from build123d import *

# Parameters (mm, degrees)
F0_W     = 60.086440295
F0_H     = 106.3739694655
F1_DEPTH = 25.4
F3_DEPTH = 12.7
F4_R     = 8.89
F4_R_2   = 5.08
F5_DEPTH = 15.24
F7_DEPTH = 12.7


with BuildPart() as f1:
    # F0 (on Top) → F1 (new body)
    with BuildSketch(Plane.XY):
        with Locations((-30.0432201475, -10.3531312197)):
            Rectangle(F0_W, F0_H)
    extrude(amount=F1_DEPTH)

    # F2 (on face) → F3 (join)
    with BuildSketch(Plane.XY.offset(25.4)):
        with BuildLine():
            ThreePointArc((-10.16, -38.1401159525), (-25.3361792847, -31.8539366677), (-19.05, -47.0301159525))
            Line((-19.05, -47.0301159525), (-19.05, -38.1401159525))
            Line((-19.05, -38.1401159525), (-10.16, -38.1401159525))
        make_face()
        with BuildLine():
            Line((-19.05, -38.1401159525), (-19.05, -47.0301159525))
            ThreePointArc((-19.05, -47.0301159525), (-12.7638207153, -44.4262952372), (-10.16, -38.1401159525))
            Line((-10.16, -38.1401159525), (-19.05, -38.1401159525))
        make_face()
        with BuildLine():
            ThreePointArc((-49.926440295, -38.1401159525), (-47.3226195797, -44.4262952372), (-41.036440295, -47.0301159525))
            Line((-41.036440295, -47.0301159525), (-41.036440295, -38.1401159525))
            Line((-41.036440295, -38.1401159525), (-49.926440295, -38.1401159525))
        make_face()
        with BuildLine():
            Line((-41.036440295, -38.1401159525), (-41.036440295, -47.0301159525))
            ThreePointArc((-41.036440295, -47.0301159525), (-34.7502610102, -44.4262952372), (-32.146440295, -38.1401159525))
            ThreePointArc((-32.146440295, -38.1401159525), (-41.036440295, -29.2501159525), (-49.926440295, -38.1401159525))
            Line((-49.926440295, -38.1401159525), (-41.036440295, -38.1401159525))
        make_face()
        with BuildLine():
            ThreePointArc((-41.036440295, 26.323853513), (-47.3226195797, 23.7200327978), (-49.926440295, 17.433853513))
            Line((-49.926440295, 17.433853513), (-41.036440295, 17.433853513))
            Line((-41.036440295, 17.433853513), (-41.036440295, 26.323853513))
        make_face()
        with BuildLine():
            Line((-41.036440295, 17.433853513), (-49.926440295, 17.433853513))
            ThreePointArc((-49.926440295, 17.433853513), (-41.036440295, 8.543853513), (-32.146440295, 17.433853513))
            ThreePointArc((-32.146440295, 17.433853513), (-34.7502610102, 23.7200327978), (-41.036440295, 26.323853513))
            Line((-41.036440295, 26.323853513), (-41.036440295, 17.433853513))
        make_face()
        with BuildLine():
            ThreePointArc((-19.05, 26.323853513), (-25.9314853388, 11.8055980522), (-10.3366687432, 15.6703460962))
            ThreePointArc((-10.3366687432, 15.6703460962), (-10.2042774497, 16.5476861679), (-10.16, 17.433853513))
            ThreePointArc((-10.16, 17.433853513), (-12.7638207153, 23.7200327978), (-19.05, 26.323853513))
        make_face()
    extrude(amount=F3_DEPTH)

    # F4 (on face) → F5 (join)
    with BuildSketch(Plane.XY.offset(25.4)):
        with Locations((-41.036440295, -38.1401159525)):
            Circle(F4_R)
        with Locations((-41.036440295, -38.1401159525)):
            Circle(F4_R_2, mode=Mode.SUBTRACT)
        with Locations((-19.05, -38.1401159525)):
            Circle(F4_R)
        with Locations((-19.05, -38.1401159525)):
            Circle(F4_R_2, mode=Mode.SUBTRACT)
        with Locations((-41.036440295, 17.433853513)):
            Circle(F4_R)
        with Locations((-41.036440295, 17.433853513)):
            Circle(F4_R_2, mode=Mode.SUBTRACT)
        with Locations((-19.05, 17.433853513)):
            Circle(F4_R)
        with Locations((-19.05, 17.433853513)):
            Circle(F4_R_2, mode=Mode.SUBTRACT)
    extrude(amount=F5_DEPTH)

    # F6 (on face) → F7 (cut)
    with BuildSketch(Plane(origin=(0, 0, 0), x_dir=(1, 0, 0), z_dir=(0, 0, -1))):
        with BuildLine():
            Line((-53.6326494753, 38.1401159525), (-48.3460910618, 38.1401159525))
            Line((-48.3460910618, 38.1401159525), (-48.3460910618, 46.6701357601))
            ThreePointArc((-48.3460910618, 46.6701357601), (-52.20384553, 43.1578080957), (-53.6326494753, 38.1401159525))
        make_face()
        with BuildLine():
            Line((-34.5826494753, 38.1401159525), (-48.3460910618, 38.1401159525))
            Line((-48.3460910618, 38.1401159525), (-53.6326494753, 38.1401159525))
            ThreePointArc((-53.6326494753, 38.1401159525), (-44.1076494753, 28.6151159525), (-34.5826494753, 38.1401159525))
        make_face()
        with BuildLine():
            Line((-48.3460910618, 46.6701357601), (-48.3460910618, 38.1401159525))
            Line((-48.3460910618, 38.1401159525), (-34.5826494753, 38.1401159525))
            ThreePointArc((-34.5826494753, 38.1401159525), (-39.0899573321, 46.2363120072), (-48.3460910618, 46.6701357601))
        make_face()
        with BuildLine():
            Line((-7.6825144947, 38.1401159525), (-26.7325144947, 38.1401159525))
            ThreePointArc((-26.7325144947, 38.1401159525), (-17.2075144947, 28.6151159525), (-7.6825144947, 38.1401159525))
        make_face()
        with BuildLine():
            ThreePointArc((-7.6825144947, 38.1401159525), (-17.2075144947, 47.6651159525), (-26.7325144947, 38.1401159525))
            Line((-26.7325144947, 38.1401159525), (-7.6825144947, 38.1401159525))
        make_face()
        with BuildLine():
            ThreePointArc((-26.7325144947, -17.433853513), (-17.2075144947, -26.958853513), (-7.6825144947, -17.433853513))
            Line((-7.6825144947, -17.433853513), (-26.7325144947, -17.433853513))
        make_face()
        with BuildLine():
            Line((-26.7325144947, -17.433853513), (-7.6825144947, -17.433853513))
            ThreePointArc((-7.6825144947, -17.433853513), (-17.2075144947, -7.908853513), (-26.7325144947, -17.433853513))
        make_face()
        with BuildLine():
            Line((-34.5826494753, -17.433853513), (-50.7258884609, -17.433853513))
            Line((-50.7258884609, -17.433853513), (-50.7258884609, -24.2840022508))
            ThreePointArc((-50.7258884609, -24.2840022508), (-40.3869708637, -26.2021016658), (-34.5826494753, -17.433853513))
        make_face()
        with BuildLine():
            Line((-50.7258884609, -17.433853513), (-53.6326494753, -17.433853513))
            ThreePointArc((-53.6326494753, -17.433853513), (-52.8758976281, -21.1545321247), (-50.7258884609, -24.2840022508))
            Line((-50.7258884609, -24.2840022508), (-50.7258884609, -17.433853513))
        make_face()
        with BuildLine():
            ThreePointArc((-34.5826494753, -17.433853513), (-44.1076494753, -7.908853513), (-53.6326494753, -17.433853513))
            Line((-53.6326494753, -17.433853513), (-50.7258884609, -17.433853513))
            Line((-50.7258884609, -17.433853513), (-34.5826494753, -17.433853513))
        make_face()
    extrude(amount=-F7_DEPTH, mode=Mode.SUBTRACT)


solid = f1.part
Check sheet for the modelled part. Datum: model origin and axes. Units: mm. A direction names the side the tool comes from. Give positions to 0.01 mm unless a question says otherwise; leave off trailing zeros. Loops run counter-clockwise (first coordinate to the right, second up) from the corner with the lowest first, then second, coordinate; pieces in that order, holes last. Notation, with made-up numbers: M 24,86 L 41,86 A13 cw 41,110 Z; hole C 77.5,-10 d8. An arc over 180 degrees is marked long. Answer as a JSON object with one key per item and string values. Group by question number.
Q1. Access from +Z, -Z, +X, -X, +Y, -Y to the whole of each face (thin tool, end or side, straight path). Record for faces 5 (the flat face through (-17, -38, 12.7)), 6 (the flat face through (-30, -10, 0)), 7 (the cylindrical face through (-10.22, 18.45, 32.91)).
Q2. Cross-section at C-C on z = 7. Record the cut outline in (x, y) (3 decimals).
Q3. Material ranges on line 1 along Y through (x, z) = (-16.5, 7); line 2 along Y through (x, z) = (-52.5, 9); line 3 along X through (y, z) = (-42.5, 11), recorded low to high. Write a range as [from, to].
Q4. Cross-section at B-B on y = 21. Record the cut outline in (x, z), then the cut area to 3 significant figures.
Q5. Cross-section at A-A on x = -37. Record the cut outline in (y, z).
Q6. Go/stop test with flat-tipped pins: P1, Ø4, axis at y = -45.5, z = 31, coming from the +X side; P2, Ø15, axis at x = -44.11, y = -38.14, coming from the -Z side; P3, Ø1.5, axis at x = -10, y = -25, coming from the -Z side; P4, Ø3, axis at x = -39.5, y = -40.5, coming from the +Z side. Record where each tip stops, or that it passes through.
Q7. Release check for a two-part mould opening along X. For faces 1 (the flat face through (-37, 14, 40.64)), 2 (the cylindrical face through (-41.62, -47.01, 32.91)), 3 (the flat face through (-60.086, -11, 13)), 4 (the flat face through (-19, 18, 38.1)) record: released by +X, released by -X, zero draft, split by the parting line, or undercut.
Q8. Cross-section at D-D on z = 28.5. Record the cut outline in (x, y).
Evaluation:
{
 "1": {"face 5": "-Z", "face 6": "-Z, +X, -X, +Y, -Y", "face 7": "+Z"},
 "2": {"outline": "M -60.086,-63.54 L 0,-63.54 L 0,42.834 L -60.086,42.834 Z; hole C -44.108,-38.14 d19.05; hole C -44.108,17.434 d19.05; hole C -17.208,-38.14 d19.05; hole C -17.208,17.434 d19.05"},
 "3": {"line 1": "y = [-63.54, -47.64], [-28.64, 7.94], [26.93, 42.83]", "line 2": "y = [-63.54, -42.65], [-33.64, 12.93], [21.94, 42.83]", "line 3": "x = [-60.09, -52.58], [-35.64, -25.68], [-8.74, 0]"},
 "4": {"outline": "M -60.09,0 L -52.94,0 L -52.94,12.7 L -35.28,12.7 L -35.28,0 L -26.04,0 L -26.04,12.7 L -8.38,12.7 L -8.38,0 L 0,0 L 0,25.4 L -10.91,25.4 L -10.91,40.64 L -15.43,40.64 L -15.43,38.1 L -22.67,38.1 L -22.67,40.64 L -27.19,40.64 L -27.19,25.4 L -32.89,25.4 L -32.89,40.64 L -37.42,40.64 L -37.42,38.1 L -44.65,38.1 L -44.65,40.64 L -49.18,40.64 L -49.18,25.4 L -60.09,25.4 Z", "area": "1,540 mm2"},
 "5": {"outline": "M -63.54,0 L -44.48,0 L -44.48,12.7 L -31.8,12.7 L -31.8,0 L 11.09,0 L 11.09,12.7 L 23.77,12.7 L 23.77,0 L 42.83,0 L 42.83,25.4 L 25.35,25.4 L 25.35,40.64 L 20.52,40.64 L 20.52,38.1 L 14.35,38.1 L 14.35,40.64 L 9.51,40.64 L 9.51,25.4 L -30.22,25.4 L -30.22,40.64 L -35.06,40.64 L -35.06,38.1 L -41.22,38.1 L -41.22,40.64 L -46.06,40.64 L -46.06,25.4 L -63.54,25.4 Z"},
 "6": {"P1": "stops at x = -11.96", "P2": "stops at z = 12.7", "P3": "stops at z = 0", "P4": "stops at z = 38.1"},
 "7": {"face 1": "zero draft", "face 2": "undercut", "face 3": "released by -X", "face 4": "undercut"},
 "8": {"outline": "C -41.04,-38.14 d17.78; C -41.04,17.43 d17.78; C -19.05,-38.14 d17.78; C -19.05,17.43 d17.78"}
}
